from build123d import *

# Parameters (mm, degrees)
SKETCH1_R           = 25
SKETCH1_R_2         = 7.5
BOSS_EXTRUDE1_DEPTH = 15


with BuildPart() as part:
    # Sketch1 → Boss-Extrude1 (new body)
    # profile 1 of 3: a face of its own
    with BuildSketch(Plane.XY):
        Circle(SKETCH1_R)
        Circle(SKETCH1_R_2, mode=Mode.SUBTRACT)
    # profile 2 of 3: a face of its own
    with BuildSketch(Plane.XY):
        with BuildLine():
            Line((-4.5, 42.591665255), (-4.5, 24.591665255))
            ThreePointArc((-4.5, 24.591665255), (0, 25), (4.5, 24.591665255))
            Line((4.5, 24.591665255), (4.5, 42.591665255))
            ThreePointArc((4.5, 42.591665255), (0, 47.091665255), (-4.5, 42.591665255))
        make_face()
    # profile 3 of 3: a face of its own
    with BuildSketch(Plane.XY):
        with BuildLine():
            Line((17.39871831, 39.1354641), (8.39871831, 23.547006832))
            ThreePointArc((8.39871831, 23.547006832), (12.5, 21.650635095), (16.192946944, 19.047006832))
            Line((16.192946944, 19.047006832), (25.192946944, 34.6354641))
            ThreePointArc((25.192946944, 34.6354641), (23.545832627, 40.782578417), (17.39871831, 39.1354641))
        make_face()
    extrude(amount=BOSS_EXTRUDE1_DEPTH)


solid = part.part
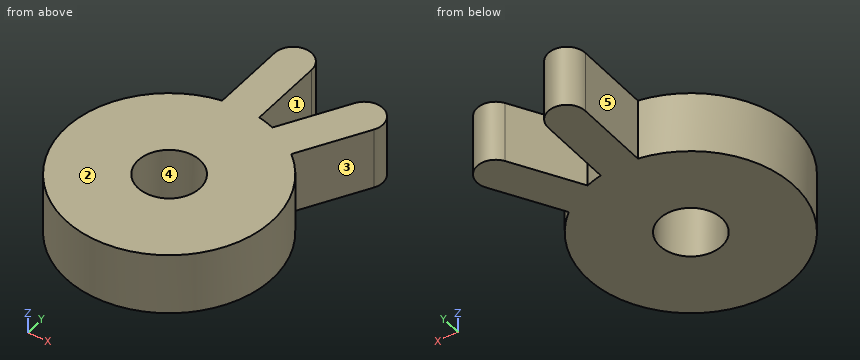
Design review of the part built by this model. Coordinates are the model's own, in mm. Face numbers are marked on the shaded views. A direction names the side the tool comes from. Coordinates: 2 decimals unless noted, no trailing zeros. Order: outer loops, then holes, each group sorted by start corner. A loop starts at its lowest first (then second) coordinate and runs counter-clockwise, first axis right, second up. Notation, with made-up numbers: (15.5, -29.5) - (68.5, -29.5) arc R29 cw to (68.5, 9.5) - close; hole circle Ø4 at (30.25, -22). An arc over 180 degrees is marked (long way). Put each result on its own line as item: value.
1) Take a section at D-D, the plane x = -18.5. Give the boundary of the cut face in (y, z).
Response values:
outline: (-16.82, 0) - (16.82, 0) - (16.82, 15) - (-16.82, 15) - close
2) Take a section at C-C, the plane z = 11.75. Give the boundary of the cut face in (x, y).
Response values:
outline: (-4.5, 24.59) arc R25 ccw (long way) to (16.19, 19.05) - (25.19, 34.64) arc R4.5 ccw to (17.4, 39.14) - (8.4, 23.55) arc R25 ccw to (4.5, 24.59) - (4.5, 42.59) arc R4.5 ccw to (-4.5, 42.59) - close; hole circle Ø15 at (0, 0)
3) Wall thickness on L1, parallel to Y at x = 0, z = 7; L2, parallel to X at y = -3, z = 4.75; L3, parallel to X at y = 6, z = 5.5: over which ranges is each line inside the solid? List them lowest first. Write a range as from..to.
Response values:
L1: y = -25..-7.5, 7.5..47.09
L2: x = -24.82..-6.87, 6.87..24.82
L3: x = -24.27..-4.5, 4.5..24.27
4) Insertion check: P1, Ø8, axis at x = 12, z = 2, coming from the -Y side; P2, Ø4, axis at x = 15, z = 12, coming from the +Y side; P3, Ø4, axis at x = -9, z = 10.5, coming from the +Y side. Each pin has a flat end and moves straight along its axis. Give the tip position at first contact, or say it passes through.
Response values:
P1: stops at y = -23.69
P2: stops at y = 38.44
P3: stops at y = 24
5) Take a section at B-B, the plane x = 0. Give the boundary of the cut face in (y, z), and give its area (3 significant figures).
Response values:
outline: (-25, 0) - (-7.5, 0) - (-7.5, 15) - (-25, 15) - close; (7.5, 0) - (47.09, 0) - (47.09, 15) - (7.5, 15) - close
area: 856 mm²
6) Tool access review of the marked faces 1 and 2: name each direction out of +Z, -Z, +X, -X, +Y, -Y from which nothing blocks a thin tool from reaching the whole face with its end or side.
Response values:
face 1: +Z, -Z, +Y
face 2: +Z, +X, -X, +Y, -Y
7) Take a section at A-A, the plane y = 0. Give the boundary of the cut face in (x, z), and give its area (3 significant figures).
Response values:
outline: (-25, 0) - (-7.5, 0) - (-7.5, 15) - (-25, 15) - close; (7.5, 0) - (25, 0) - (25, 15) - (7.5, 15) - close
area: 525 mm²
8) The part is to be moulded in two halves that separate along X. For the marked faces 3, 4 and 5, say which applies: released by +X, released by -X, zero draft, split by the parting line, or undercut.
Response values:
face 3: released by +X
face 4: undercut
face 5: released by -X
